```python
from build123d import *

# Parameters (mm, degrees)
BOSS_EXTRUDE1_DEPTH = 59.94146
SKETCH2_R           = 8.099936755
BOSS_EXTRUDE2_DEPTH = 6.09219
BOSS_EXTRUDE3_START = 25.228296
SKETCH2_2_R         = 8.099936755
BOSS_EXTRUDE3_DEPTH = 6.09219


with BuildPart() as part:
    # Sketch1 → Boss-Extrude1 (new body)
    with BuildSketch(Plane(origin=(80.083152, 0, 0), x_dir=(0, 0, -1), z_dir=(1, 0, 0))):
        Polygon((267.4874, 138.173968), (272.174462, 159.761428), (368.557048, 108.729526), (342.20531, 98.6155), align=None)
    extrude(amount=BOSS_EXTRUDE1_DEPTH)

    # Sketch2 → Boss-Extrude2 (add)
    with BuildSketch(Plane(origin=(87.778844, 0, 0), x_dir=(0, 0, -1), z_dir=(1, 0, 0))):
        with BuildLine():
            Line((271.238218, 136.721088), (266.19327, 112.593374))
            ThreePointArc((266.19327, 112.593374), (271.461683784, 96.939756218), (287.369758, 101.381052))
            Line((287.369758, 101.381052), (304.489612, 119.115332))
            Line((304.489612, 119.115332), (271.238218, 136.721088))
        make_face()
        with Locations(Location((275.620988, 106.805984, 0), (0, 0, 180))):
            Circle(SKETCH2_R, mode=Mode.SUBTRACT)
    extrude(amount=BOSS_EXTRUDE2_DEPTH)

    # Sketch2<2> → Boss-Extrude3 (add)
    with BuildSketch(Plane(origin=(87.778844, 0, 0), x_dir=(0, 0, -1), z_dir=(1, 0, 0)).offset(BOSS_EXTRUDE3_START)):
        with BuildLine():
            Line((271.238218, 136.721088), (266.19327, 112.593374))
            ThreePointArc((266.19327, 112.593374), (271.461683784, 96.939756218), (287.369758, 101.381052))
            Line((287.369758, 101.381052), (304.489612, 119.115332))
            Line((304.489612, 119.115332), (271.238218, 136.721088))
        make_face()
        with Locations(Location((275.620988, 106.805984, 0), (0, 0, 180))):
            Circle(SKETCH2_2_R, mode=Mode.SUBTRACT)
    extrude(amount=BOSS_EXTRUDE3_DEPTH)


solid = part.part
```
Could you check a few things on this model? Use its own coordinates, in mm. A direction names the side the tool comes from. Coordinates: 2 decimals unless noted, no trailing zeros. Write each loop counter-clockwise with the first axis right and the second up, starting at its lowest first coordinate (ties: lowest second). Pieces come first, ordered by that corner, then holes. Notation, with made-up numbers: (77, 3.5) -> (107, 3.5) arc R11 ccw to (107, 24.5) -> close; hole circle Ø5 at (63, -9). An arc over 180 degrees is marked (long way). Return JSON: item names as keys, results as strings.
(1) I need wall thicknesses on L1, parallel to X at y = 122.5, z = -275.5; L2, parallel to Z at x = 113.5, y = 111; L3, parallel to Y at x = 110, z = -282. Which ranges of each line are inside material? Lowest first, please.
Numbers:
{"L1": "x = 87.78 to 93.87, 113.01 to 119.1", "L2": "z = -364.27 to -318.81, -296.66 to -282.55, -268.69 to -265.59", "L3": "y = 130.49 to 154.56"}
(2) Imagine slicing it at B-B, the plane y = 116. Please give me the cut outline in (x, z).
Numbers:
{"outline": "(80.08, -354.83) -> (140.02, -354.83) -> (140.02, -309.37) -> (80.08, -309.37) -> close; (87.78, -301.48) -> (93.87, -301.48) -> (93.87, -266.91) -> (87.78, -266.91) -> close; (113.01, -301.48) -> (119.1, -301.48) -> (119.1, -266.91) -> (113.01, -266.91) -> close"}
(3) Imagine slicing it at A-A, the plane x = 116.5. Please give me the cut outline in (y, z), then the cut area to 3 significant figures.
Numbers:
{"outline": "(98.62, -342.21) -> (108.73, -368.56) -> (159.76, -272.17) -> (138.17, -267.49) -> (136.24, -271.14) -> (112.59, -266.19) arc R12 ccw to (101.38, -287.37) -> (118.76, -304.15) -> close; hole circle Ø16.2 at (106.81, -275.62)", "area": "2,780 mm2"}
(4) Imagine slicing it at D-D, the plane z = -288.5. Please give me the cut outline in (x, y).
Numbers:
{"outline": "(80.08, 127.05) -> (87.78, 127.05) -> (87.78, 102.55) -> (93.87, 102.55) -> (93.87, 127.05) -> (113.01, 127.05) -> (113.01, 102.55) -> (119.1, 102.55) -> (119.1, 127.05) -> (140.02, 127.05) -> (140.02, 151.12) -> (80.08, 151.12) -> close"}
(5) I'm going to push flat-ended pins straight in: pin 1 (2 mm diameter, centred on x = 87, z = -304, fed in from -Y); pin 2 (5 mm diameter, centred on x = 108.5, y = 113, fed in from -Z); pin 3 (10 mm diameter, centred on y = 117.5, z = -282, fed in from -X); pin 4 (12 mm diameter, centred on y = 112, z = -312.5, fed in from +X). Where does each tip first touch, or does it pass through?
Numbers:
{"pin 1": "stops at y = 117.96", "pin 2": "stops at z = -365.21", "pin 3": "stops at x = 87.78", "pin 4": "stops at x = 140.02"}
(6) Imagine slicing it at C-C, the plane y = 103.5. Please give me the cut outline in (x, z).
Numbers:
{"outline": "(80.08, -354.93) -> (140.02, -354.93) -> (140.02, -332.98) -> (80.08, -332.98) -> close; (87.78, -289.42) -> (93.87, -289.42) -> (93.87, -283.02) -> (87.78, -283.02) -> close; (87.78, -268.23) -> (93.87, -268.23) -> (93.87, -265.78) -> (87.78, -265.78) -> close; (113.01, -289.42) -> (119.1, -289.42) -> (119.1, -283.02) -> (113.01, -283.02) -> close; (113.01, -268.23) -> (119.1, -268.23) -> (119.1, -265.78) -> (113.01, -265.78) -> close"}
(7) We'd pull the mould along Y, two halves only. Please class faces 6 (the flat face through (80.083, 127, -315)), 7 (the cylindrical face through (116.01, 109.91, -268.14)), 8 (the flat face through (90.78, 109.95, -295.64)), 9 (the flat face through (116.01, 124.58, -268.7)): +Y half, -Y half, draft (parallel to the pull), parting line (faces both ways), or undercut.
Numbers:
{"face 6": "draft", "face 7": "undercut", "face 8": "-Y half", "face 9": "undercut"}
(8) Which directions (+Z, -Z, +X, -X, +Y, -Y) give clear straight access to the entire face, cutting with the end or side of a thin tool? Please do faces 1 (the flat face through (87.779, 116, -280)), 2 (the flat face through (116.01, 109.95, -295.64)), 3 (the flat face through (90.78, 124.58, -268.7)), 4 (the flat face through (113.007, 116, -280)), 5 (the flat face through (119.099, 116, -280)).
Numbers:
{"face 1": "+Z, -X, -Y", "face 2": "+X, -X, -Y", "face 3": "+Z, +X, -X", "face 4": "+Z, -Y", "face 5": "+Z, +X, -Y"}
